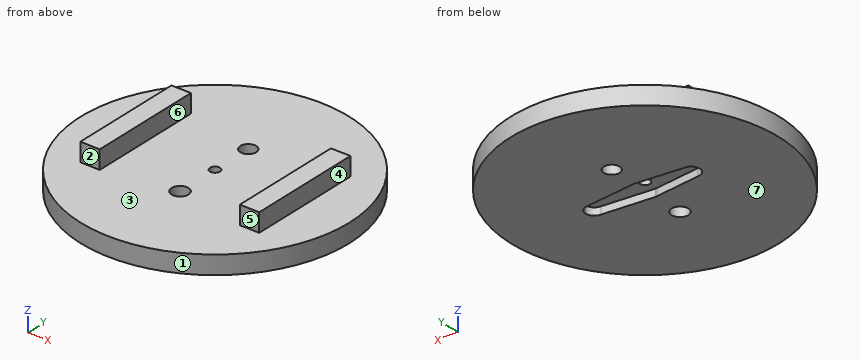
```python
from build123d import *

# Parameters (mm, degrees)
F0_R     = 36.3144122586
F3_DEPTH = 5
F1_W     = 5.236171186
F1_H     = 30.8128492907
F4_DEPTH = 10
F2_R     = 2.2829264836
F2_R_2   = 1.3509728807
F2_R_3   = 2.1549795906
F5_DEPTH = 25
F7_DEPTH = 2


with BuildPart() as f3:
    # F0 (on Top) → F3 (new body)
    with BuildSketch(Plane.XY):
        Circle(F0_R)
    extrude(amount=F3_DEPTH)

    # F1 (on Top) → F4 (join)
    with BuildSketch(Plane.XY):
        with Locations((21.547390148, 0.1232274808)):
            Rectangle(F1_W, F1_H)
        Polygon((-24.165475741, 15.5296521261), (-24.165475741, 0), (-24.165475741, -15.2831971645), (-18.9293045551, -15.2831971645), (-18.9293045551, 15.5296521261), align=None)
    extrude(amount=F4_DEPTH)

    # F2 (on Top) → F5 (cut)
    with BuildSketch(Plane.XY):
        with Locations((0, -11.8196206167)):
            Circle(F2_R)
        Circle(F2_R_2)
        with Locations((0, 11.250000447)):
            Circle(F2_R_3)
    extrude(amount=F5_DEPTH, mode=Mode.SUBTRACT)

    # F6 (on Top) → F7 (cut)
    with BuildSketch(Plane.XY):
        with BuildLine():
            ThreePointArc((-0.3703859768, -3.5693595734), (2.402953818, -2.6652066495), (3.5885252592, 0))
            ThreePointArc((3.5885252592, 0), (2.402953818, 2.6652066495), (-0.3703859768, 3.5693595734))
            ThreePointArc((-0.3703859768, 3.5693595734), (-3.5885252592, 0), (-0.3703859768, -3.5693595734))
        make_face()
        with BuildLine():
            ThreePointArc((-0.3703859768, 3.5693595734), (2.402953818, 2.6652066495), (3.5885252592, 0))
            ThreePointArc((3.5885252592, 0), (2.402953818, -2.6652066495), (-0.3703859768, -3.5693595734))
            Line((-0.3703859768, -3.5693595734), (0, -3.6077938568))
            Line((0, -3.6077938568), (13.7103013694, -2.3183212426))
            ThreePointArc((13.7103013694, -2.3183212426), (11.3919801268, 0), (13.7103013694, 2.3183212426))
            Line((13.7103013694, 2.3183212426), (0, 3.6077938568))
            Line((0, 3.6077938568), (-0.3703859768, 3.5693595734))
        make_face()
        with BuildLine():
            ThreePointArc((-0.3703859768, -3.5693595734), (-3.5885252592, 0), (-0.3703859768, 3.5693595734))
            Line((-0.3703859768, 3.5693595734), (-12.5144906342, 2.3091877811))
            ThreePointArc((-12.5144906342, 2.3091877811), (-10.8816482952, 1.632842339), (-10.2053028531, 0))
            ThreePointArc((-10.2053028531, 0), (-10.8816482952, -1.632842339), (-12.5144906342, -2.3091877811))
            Line((-12.5144906342, -2.3091877811), (-0.3703859768, -3.5693595734))
        make_face()
        with BuildLine():
            Line((-12.5144906342, 0), (-12.5144906342, 2.3091877811))
            ThreePointArc((-12.5144906342, 2.3091877811), (-14.8236784153, 0), (-12.5144906342, -2.3091877811))
            Line((-12.5144906342, -2.3091877811), (-12.5144906342, 0))
        make_face()
        with BuildLine():
            ThreePointArc((-10.2053028531, 0), (-10.8816482952, 1.632842339), (-12.5144906342, 2.3091877811))
            Line((-12.5144906342, 2.3091877811), (-12.5144906342, 0))
            Line((-12.5144906342, 0), (-12.5144906342, -2.3091877811))
            ThreePointArc((-12.5144906342, -2.3091877811), (-10.8816482952, -1.632842339), (-10.2053028531, 0))
        make_face()
        with BuildLine():
            Line((13.7103013694, 0), (13.7103013694, 2.3183212426))
            ThreePointArc((13.7103013694, 2.3183212426), (11.3919801268, 0), (13.7103013694, -2.3183212426))
            Line((13.7103013694, -2.3183212426), (13.7103013694, 0))
        make_face()
        with BuildLine():
            ThreePointArc((16.0286226121, 0), (15.3496020411, 1.6393006716), (13.7103013694, 2.3183212426))
            Line((13.7103013694, 2.3183212426), (13.7103013694, 0))
            Line((13.7103013694, 0), (13.7103013694, -2.3183212426))
            ThreePointArc((13.7103013694, -2.3183212426), (15.3496020411, -1.6393006716), (16.0286226121, 0))
        make_face()
    extrude(amount=F7_DEPTH, mode=Mode.SUBTRACT)


solid = f3.part
```
Could you check a few things on this model? Use its own coordinates, in mm. Face numbers are marked on the shaded views. A direction names the side the tool comes from. Give positions to 0.01 mm unless a question says otherwise; leave off trailing zeros. Loops run counter-clockwise (first coordinate to the right, second up) from the corner with the lowest first, then second, coordinate; pieces in that order, holes last. Notation, with made-up numbers: (48.5, -16.5) - (52.5, -16.5) arc R31 cw to (52.5, 19.5) - close; hole circle Ø9 at (-23.5, 62.5). An arc over 180 degrees is marked (long way). Use one line per item in the form item = value.
1. On a 3-axis mill with a long thin cutter (end or side, diameter ignored), from which of +Z, -Z, +X, -X, +Y, -Y can I reach the whole of each face in a straight line? I mean the marked faces 5, 6 and 7. Say none if no direction works.
Response values:
face_5 = +Z, +X, -X, -Y
face_6 = +Z, +Y, -Y
face_7 = -Z, +X, -X, +Y, -Y
2. I want a section at C-C (x = 10.5). Please give me the cut outline in (y, z), and give its area (3 significant figures).
Response values:
outline = (-34.76, 0) - (-2.62, 0) - (-2.62, 2) - (2.62, 2) - (2.62, 0) - (34.76, 0) - (34.76, 5) - (-34.76, 5) - close
area = 337 mm²
3. I want a section at D-D (z = 3). Please give me the cut outline in (x, y).
Response values:
outline = circle Ø72.63 at (0, 0); hole circle Ø4.57 at (0, -11.82); hole circle Ø4.31 at (0, 11.25); hole circle Ø2.7 at (0, 0)
4. I want a section at A-A (z = 6.75). Please give me the cut outline in (x, y), and give its area (3 significant figures).
Response values:
outline = (-24.17, -15.28) - (-18.93, -15.28) - (-18.93, 15.53) - (-24.17, 15.53) - close; (18.93, -15.28) - (24.17, -15.28) - (24.17, 15.53) - (18.93, 15.53) - close
area = 323 mm²
5. I want a section at B-B (y = 12.5). Please give me the cut outline in (x, z), and give its area (3 significant figures).
Response values:
outline = (-34.1, 0) - (-1.76, 0) - (-1.76, 5) - (-18.93, 5) - (-18.93, 10) - (-24.17, 10) - (-24.17, 5) - (-34.1, 5) - close; (1.76, 0) - (34.1, 0) - (34.1, 5) - (24.17, 5) - (24.17, 10) - (18.93, 10) - (18.93, 5) - (1.76, 5) - close
area = 376 mm²
6. I'm going to push flat-ended pins straight in: pin 1 Ø6 at (x, z) = (-21.5, 7.5) entering from -Y; pin 2 Ø5.5 at (x, z) = (-20.5, 8.5) entering from -Y; pin 3 Ø5.5 at (x, y) = (0, -11.82) entering from +Z; pin 4 Ø1.6 at (x, y) = (0, 0) entering from +Z. Where does each tip first touch, or does it pass through?
Response values:
pin_1 = -30.41
pin_2 = -15.28
pin_3 = 5
pin_4 = through
7. Thinking about a two-plate mould opening in X: for the marked faces 1, 2, 3 and 4, which applies, released by +X, released by -X, zero draft, split by the parting line, or undercut?
Response values:
face_1 = split by the parting line
face_2 = zero draft
face_3 = undercut
face_4 = released by +X
8. I need wall thicknesses on probe 1 along Y at (x, z) = (0, 4.35); probe 2 along Y at (x, z) = (0, 1.7); probe 3 along Z at (x, y) = (15.5, 24). Which ranges of each line are inside material? Lowest first, please.
Response values:
probe_1 = -36.31 to -14.1, -9.54 to -1.35, 1.35 to 9.1, 13.4 to 36.31
probe_2 = -36.31 to -14.1, -9.54 to -3.61, 3.61 to 9.1, 13.4 to 36.31
probe_3 = 0 to 5
